For this review, take the finished solid that the model builds, in its own axes (mm). A direction names the side the tool comes from. Coordinates: 2 decimals unless noted, no trailing zeros. Order: outer loops, then holes, each group sorted by start corner. A loop starts at its lowest first (then second) coordinate and runs counter-clockwise, first axis right, second up.
from build123d import *

# Parameters (mm, degrees)
SKETCH1_R           = 3.25
BOSS_EXTRUDE1_DEPTH = 22.5
SKETCH2_R           = 1.5
CUT_EXTRUDE1_DEPTH  = 15
SKETCH3_R           = 5
BOSS_EXTRUDE2_DEPTH = 5


with BuildPart() as part:
    # Sketch1 → Boss-Extrude1 (new, symmetric)
    with BuildSketch(Plane(origin=(0, 0, 0), x_dir=(0, 0, -1), z_dir=(1, 0, 0))):
        with Locations(Location((0, 0, 0), (0, 0, 180))):
            Circle(SKETCH1_R)
    extrude(amount=BOSS_EXTRUDE1_DEPTH, both=True)

    # Sketch2 → Cut-Extrude1 (cut, symmetric)
    with BuildSketch(Plane.XY):
        with Locations((-19.5, 0)):
            Circle(SKETCH2_R)
        with Locations((19.5, 0)):
            Circle(SKETCH2_R)
    extrude(amount=CUT_EXTRUDE1_DEPTH, both=True, mode=Mode.SUBTRACT)

    # Sketch3 → Boss-Extrude2 (add, symmetric)
    with BuildSketch(Plane(origin=(0, 0, 0), x_dir=(0, 0, -1), z_dir=(1, 0, 0))):
        Circle(SKETCH3_R)
    extrude(amount=BOSS_EXTRUDE2_DEPTH, both=True)


solid = part.part
1. To check wall thickness, follow L1, parallel to X at y = 0, z = -1.5; L2, parallel to Y at x = -19.5, z = 2.3; L3, parallel to Z at x = -8.5, y = 0.25. State the ranges of each line that lie inside material, in increasing order.
Answer below:
L1: x = -22.5 to -21, -18 to 18, 21 to 22.5
L2: y = -2.3 to -1.5, 1.5 to 2.3
L3: z = -3.24 to 3.24
2. Machinability: for faces 1 (the face through (22.5, 0, 0)), 2 (the face through (5, -3.3, -1)), 3 (the face through (-5, -3.3, -1)), which of the approach directions +Z, -Z, +X, -X, +Y, -Y give a long, thin tool a straight path to every point of the face, cutting with its end or side? Answer none if there is none.
Answer below:
face 1: +Z, -Z, +X, +Y, -Y
face 2: +X
face 3: -X
3. Clearance check with flat-ended pins moving along their axes: pin 1 Ø2.5 at (x, y) = (19.5, 0) entering from -Z; pin 2 Ø6 at (x, y) = (7, -2.5) entering from -Z; pin 3 Ø1.5 at (x, y) = (15, -0.5) entering from -Z; pin 4 Ø4 at (x, y) = (-19.5, 0) entering from +Z. State where each tip first meets the part, or that it passes through.
Answer below:
pin 1: passes through
pin 2: stops at z = -4.99
pin 3: stops at z = -3.25
pin 4: stops at z = 3.25
4. Take a section at C-C, the plane y = -2. Give the boundary of the cut face in (x, z).
Answer below:
outline: (-22.5, -2.56) - (-5, -2.56) - (-5, -4.58) - (5, -4.58) - (5, -2.56) - (22.5, -2.56) - (22.5, 2.56) - (5, 2.56) - (5, 4.58) - (-5, 4.58) - (-5, 2.56) - (-22.5, 2.56) - close
5. Take a section at D-D, the plane x = 19.5. Give the boundary of the cut face in (y, z).
Answer below:
outline: (-1.5, -2.88) - (-1.5, 2.88) arc R3.25 ccw to start; (1.5, -2.88) arc R3.25 ccw to (1.5, 2.88) - close
6. Take a section at B-B, the plane x = 10. Give the boundary of the cut face in (y, z), plus the area to 3 significant figures.
Answer below:
outline: circle Ø6.5 at (0, 0)
area: 33.2 mm2
7. The part is to be moulded in two halves that separate along Y. For faces 4 (the face through (-22.5, 0, 0)), 5 (the face through (-13.628, -0.143, -3.247)), 6 (the face through (21, 0, 0)), say which applies: +Y half, -Y half, draft (parallel to the pull), parting line (faces both ways), or undercut.
Answer below:
face 4: draft
face 5: parting line
face 6: undercut
8. Take a section at A-A, the plane z = 1.75. Give the boundary of the cut face in (x, y), plus the area to 3 significant figures.
Answer below:
outline: (-22.5, -2.74) - (-5, -2.74) - (-5, -4.68) - (5, -4.68) - (5, -2.74) - (22.5, -2.74) - (22.5, 2.74) - (5, 2.74) - (5, 4.68) - (-5, 4.68) - (-5, 2.74) - (-22.5, 2.74) - close; hole circle Ø3 at (-19.5, 0); hole circle Ø3 at (19.5, 0)
area: 271 mm2
